Model file for the job. Use its own axes, mm. A direction names the side the tool comes from. Round coordinates to 2 decimals unless told otherwise and drop trailing zeros. Write each loop counter-clockwise with the first axis right and the second up, starting at its lowest first coordinate (ties: lowest second). Pieces come first, ordered by that corner, then holes.
```python
from build123d import *

# Parameters (mm, degrees)
SKETCH1_R           = 9.25
BOSS_EXTRUDE1_DEPTH = 3


with BuildPart() as part:
    # Sketch1 → Boss-Extrude1 (new body)
    with BuildSketch(Plane.XY):
        Polygon((10, -22.5), (62, -22.5), (62, -10), (65, -10), (65, 10), (62, 10), (62, 22.5), (38.3, 22.5), (38.3, 19.5), (39.65, 19.5), (39.65, 17), (38.3, 17), (38.3, 12.5), (35, 12.5), (35, 17), (33.65, 17), (33.65, 19.5), (35, 19.5), (35, 22.5), (10, 22.5), (10, 25.5), (-10, 25.5), (-10, 22.5), (-35, 22.5), (-35, 19.5), (-33.65, 19.5), (-33.65, 17), (-35, 17), (-35, 12.5), (-38.3, 12.5), (-38.3, 17), (-39.65, 17), (-39.65, 19.5), (-38.3, 19.5), (-38.3, 22.5), (-62, 22.5), (-62, 10), (-65, 10), (-65, -10), (-62, -10), (-62, -22.5), (-10, -22.5), (-10, -25.5), (10, -25.5), align=None)
        with Locations((-12.75, -7.5)):
            Circle(SKETCH1_R, mode=Mode.SUBTRACT)
        with BuildLine():
            ThreePointArc((-3.5, -18.5), (-6, -16), (-3.5, -13.5))
            Line((-3.5, -13.5), (3.5, -13.5))
            ThreePointArc((3.5, -13.5), (6, -16), (3.5, -18.5))
            Line((3.5, -18.5), (-3.5, -18.5))
        make_face(mode=Mode.SUBTRACT)
        with Locations((12.75, -7.5)):
            Circle(SKETCH1_R, mode=Mode.SUBTRACT)
        with BuildLine():
            ThreePointArc((6, 0.5), (5.414213562, -0.914213562), (4, -1.5))
            Line((4, -1.5), (-4, -1.5))
            ThreePointArc((-4, -1.5), (-5.414213562, -0.914213562), (-6, 0.5))
            Line((-6, 0.5), (-6, 1.5))
            Line((-6, 1.5), (6, 1.5))
            Line((6, 1.5), (6, 0.5))
        make_face(mode=Mode.SUBTRACT)
    extrude(amount=BOSS_EXTRUDE1_DEPTH)


solid = part.part
```
1) Cut at D-D on x = -24.5. List the corners of the cut face in (y, z).
2) Cut at C-C on y = -20. List the corners of the cut face in (x, z).
3) Wall check: probe 1 along Y at (x, z) = (-1.5, 2.05); probe 2 along X at (y, z) = (21.5, 0.25); probe 3 along Y at (x, z) = (-12.75, 0.6). Give the ranges that are in metal, low to high.
4) Cut at B-B on y = -7.5. List the corners of the cut face in (x, z), and give its area (3 significant figures).
5) Cut at A-A on x = 12.75. List the corners of the cut face in (y, z), and give its area (3 significant figures).
6) Pull direction X, two halves, no side cores. Call faces 1 (the face through (-1, -5, 3)), 2 (the face through (-65, 0, 1)), 3 (the face through (-6, -16, 1)): released by +X, released by -X, zero draft, split by the parting line, or undercut.
7) Flat gauge pins, fed straight in: pin 1 Ø12 at (x, y) = (15, -7.5) entering from +Z; pin 2 Ø1.5 at (y, z) = (20.5, 1) entering from -X; pin 3 Ø0.9 at (x, z) = (-39.5, 2) entering from -Y; pin 4 Ø1.5 at (y, z) = (14.5, 1.5) entering from +X. Where does each tip first touch, or does it go through?
8) Which spindle directions (+Z, -Z, +X, -X, +Y, -Y) get a long thin tool onto all of the face, cutting with end or side? Do faces 4 (the face through (35, 15, 1)), 5 (the face through (-50, 22.5, 1)), 6 (the face through (63, -10, 1)), 7 (the face through (-36, -22.5, 1)), 8 (the face through (64, 10, 1)). Say none if no direction does.
Result sheet:
1. outline: (-22.5, 0) - (22.5, 0) - (22.5, 3) - (-22.5, 3) - close
2. outline: (-62, 0) - (62, 0) - (62, 3) - (-62, 3) - close
3. probe 1: y = -25.5 to -18.5, -13.5 to -1.5, 1.5 to 25.5
3. probe 2: x = -62 to -38.3, -35 to 35, 38.3 to 62
3. probe 3: y = -22.5 to -16.75, 1.75 to 22.5
4. outline: (-65, 0) - (-22, 0) - (-22, 3) - (-65, 3) - close; (-3.5, 0) - (3.5, 0) - (3.5, 3) - (-3.5, 3) - close; (22, 0) - (65, 0) - (65, 3) - (22, 3) - close
4. area: 279 mm2
5. outline: (-22.5, 0) - (-16.75, 0) - (-16.75, 3) - (-22.5, 3) - close; (1.75, 0) - (22.5, 0) - (22.5, 3) - (1.75, 3) - close
5. area: 79.5 mm2
6. face 1: zero draft
6. face 2: released by -X
6. face 3: undercut
7. pin 1: passes through
7. pin 2: stops at x = -62
7. pin 3: stops at y = -22.5
7. pin 4: stops at x = 62
8. face 4: +Z, -Z, +Y
8. face 5: +Z, -Z, -X, +Y
8. face 6: +Z, -Z, +X, -Y
8. face 7: +Z, -Z, -X, -Y
8. face 8: +Z, -Z, +X, +Y
